Solid Edge part; units mm, degrees
sketch "Sketch1" plane through (0, 0, 0) normal (1, 0, 0) x (0, 1, 0)
  arc A0 (28.4759, 67.4357) -> (25.3647, 67.4357) centre (26.9203, 65.8801) ccw
  line L0 (25.3647, 67.4357) -> (0.659, 42.7301)
  arc A1 (0.659, 42.7301) -> (0, 41.1391) centre (2.25, 41.1391) ccw
  line L1 (0, 41.1391) -> (0, 40)
  line L2 (0, 40) -> (0, 0)
  line L3 (0, 0) -> (5, 0)
  line L4 (5, 0) -> (5, 27.75)
  arc A2 (5, 27.75) -> (7.25, 30) centre (7.25, 27.75) cw
  line L5 (7.75, 30) -> (7.25, 30)
  arc A3 (10, 27.75) -> (7.75, 30) centre (7.75, 27.75) ccw
  line L6 (10, 27.75) -> (10, 0)
  line L7 (10, 0) -> (15, 0)
  line L8 (15, 0) -> (15, 32.8)
  arc A4 (12.8, 35) -> (15, 32.8) centre (12.8, 32.8) cw
  line L9 (7.2, 35) -> (12.8, 35)
  line L10 (7.2, 35) -> (10, 35)
  arc A5 (5, 37.2) -> (7.2, 35) centre (7.2, 37.2) ccw
  line L11 (5, 38.985) -> (5, 37.2)
  arc A6 (5.7177, 40.7177) -> (5, 38.985) centre (7.4505, 38.985) ccw
  line L12 (5.7177, 40.7177) -> (28.9002, 63.9002)
  arc A7 (28.9002, 63.9002) -> (28.9002, 67.0115) centre (27.3446, 65.4558) ccw
  line L13 (28.9002, 67.0115) -> (28.4759, 67.4357)
extrude "Protrusion1" add sketch "Sketch1" against normal blind 86 material side at (0, 26.9203, 68.1301)
sketch "Sketch2" plane through (-43, 13.0118, 55.0829) normal (0, -0.7071068, 0.7071068) x (1, 0, 0)
  line L0 (38, -13) -> (38, 13)
  line L1 (38, 13) -> (-38, 13)
  line L2 (-38, 13) -> (-38, -13)
  line L3 (-38, -13) -> (38, -13)
extrude "Cutout1" cut sketch "Sketch2" against normal blind 5
Work out the finished part from the listing and answer in its coordinate system (mm). A direction names the side the tool comes from. Give positions to 0.01 mm unless a question says otherwise; leave off trailing zeros. Loops run counter-clockwise (first coordinate to the right, second up) from the corner with the lowest first, then second, coordinate; pieces in that order, holes last. Notation, with made-up numbers: (21, -25) - (74, -25) arc R29 cw to (74, 4) - close; hole circle Ø2 at (-35.5, -31.75). An arc over 180 degrees is marked (long way). Answer in a Markdown table with one row per item. Add a question column.
Q1. The part is cut by section D-D (y = 19). Determine the outline of the cut face in (x, z), and give its area (3 significant figures).
Q2. Consider line 1 along Y through (x, z) = (-6.5, 26.5); line 2 along X through (y, z) = (10.25, 47.5); line 3 along Z through (x, y) = (-81.5, 8.75). Determine where each line is inside the solid, lowest interval first.
Q3. The part is cut by section A-A (z = 25). Determine the outline of the cut face in (x, y).
Q4. The part is cut by section C-C (y = 11). Determine the outline of the cut face in (x, z).
Q5. Determine the mould class of faces 1 (the flat face through (-5, 15, 53)), 2 (the flat face through (-86, 11, 26)), 3 (the cylindrical face through (-42.398, 29.544, 65.432)) for opening direction X: released by +X, released by -X, zero draft, split by the parting line, or undercut.
Q6. Each of these flat-tipped pins is pushed along its axis until it touches: P1, Ø3, axis at x = -60, z = 35, coming from the +Y side; P2, Ø8.5, axis at x = -32, z = 9, coming from the +Y side; P3, Ø1.5, axis at x = -42, y = 13.5, coming from the +Z side; P4, Ø10, axis at x = -17, z = 55.5, coming from the +Y side. Where does it stop, or does it pass through?
Q7. A tool of negligible diameter and unlimited length cuts with its end or side. For faces 4 (the cylindrical face through (-42.4, 26.94, 68.08)), 5 (the cylindrical face through (-42.398, 5.192, 39.935)), 6 (the flat face through (-45.985, 23.135, 65.206)), 7 (the flat face through (-42.47, 23.95, 62.53)), 8 (the flat face through (-42, 10, 14)), from which of +Z, -Z, +X, -X, +Y, -Y can it reach the whole face along a straight path? Write none if from no direction.
Solution:
| question | item | result |
|---|---|---|
| 1 | outline | (-86, 54) - (-81, 54) - (-81, 61.07) - (-86, 61.07) - close; (-5, 54) - (0, 54) - (0, 61.07) - (-5, 61.07) - close |
| 1 | area | 70.7 mm² |
| 2 | line 1 | y = 0 to 5, 10 to 15 |
| 2 | line 2 | x = -86 to -81, -5 to 0 |
| 2 | line 3 | z = 29.77 to 35, 43.75 to 50.82 |
| 3 | outline | (-86, 0) - (0, 0) - (0, 5) - (-86, 5) - close; (-86, 10) - (0, 10) - (0, 15) - (-86, 15) - close |
| 4 | outline | (-86, 0) - (0, 0) - (0, 35) - (-86, 35) - close; (-86, 46) - (-81, 46) - (-81, 53.07) - (-86, 53.07) - close; (-5, 46) - (0, 46) - (0, 53.07) - (-5, 53.07) - close |
| 5 | face 1 | undercut |
| 5 | face 2 | released by -X |
| 5 | face 3 | zero draft |
| 6 | P1 | stops at y = 14.89 |
| 6 | P2 | stops at y = 15 |
| 6 | P3 | stops at z = 35 |
| 6 | P4 | passes through |
| 7 | face 4 | +Z, +X, -X |
| 7 | face 5 | +X, -X, +Y |
| 7 | face 6 | +Z, +X, -X, -Y |
| 7 | face 7 | -Z, -Y |
| 7 | face 8 | -Z, +X, -X |
